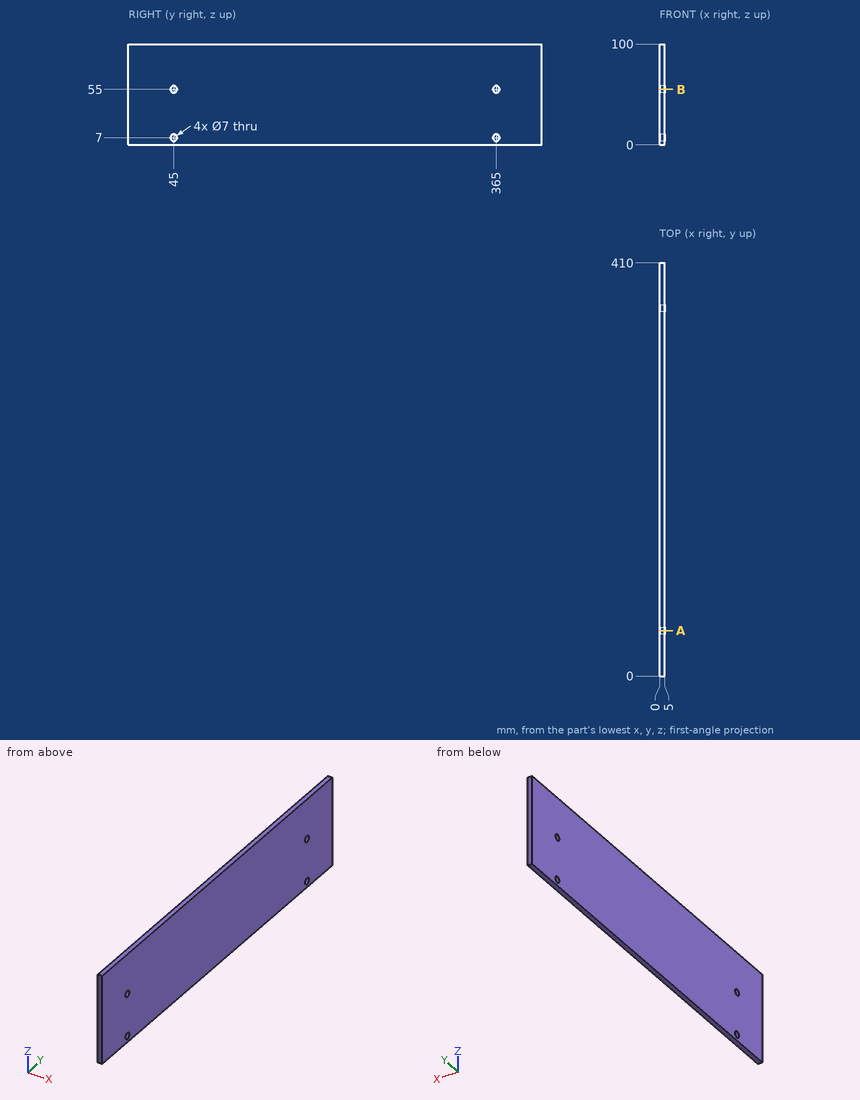
Answer from the drawing. Dimensions are ordinates in mm from the lowest x, y and z of the part. Coordinates: 2 decimals unless noted, no trailing zeros. Write each loop counter-clockwise with the first axis right and the second up, starting at its lowest first coordinate (ties: lowest second). Pieces come first, ordered by that corner, then holes. Notation, with made-up numbers: M -0.75,19.5 L 26.25,19.5 A16 cw 26.25,47.5 Z; hole C -39,1 d5. An arc over 180 degrees is marked long. Put each result on its own line as item: value. Start each with the question number.
1. A cutting plane is placed at A-A on y = 45. Write down the section's boundary in (x, z), then the cut area to 3 significant figures.
2. Consider line 1 (Z direction, x = 1.25, y = 365). Determine where the line is inside the solid, lowest interval first. Write a range as from..to.
3. A cutting plane is placed at B-B on z = 55. Write down the section's boundary in (x, y), then the cut area to 3 significant figures.
Resolved:
1. outline: M 0,0 L 5,0 L 5,3.5 L 0,3.5 Z; M 0,10.5 L 5,10.5 L 5,51.5 L 0,51.5 Z; M 0,58.5 L 5,58.5 L 5,100 L 0,100 Z
1. area: 430 mm2
2. line 1: z = 0..3.5, 10.5..51.5, 58.5..100
3. outline: M 0,0 L 5,0 L 5,41.5 L 0,41.5 Z; M 0,48.5 L 5,48.5 L 5,361.5 L 0,361.5 Z; M 0,368.5 L 5,368.5 L 5,410 L 0,410 Z
3. area: 1,980 mm2
